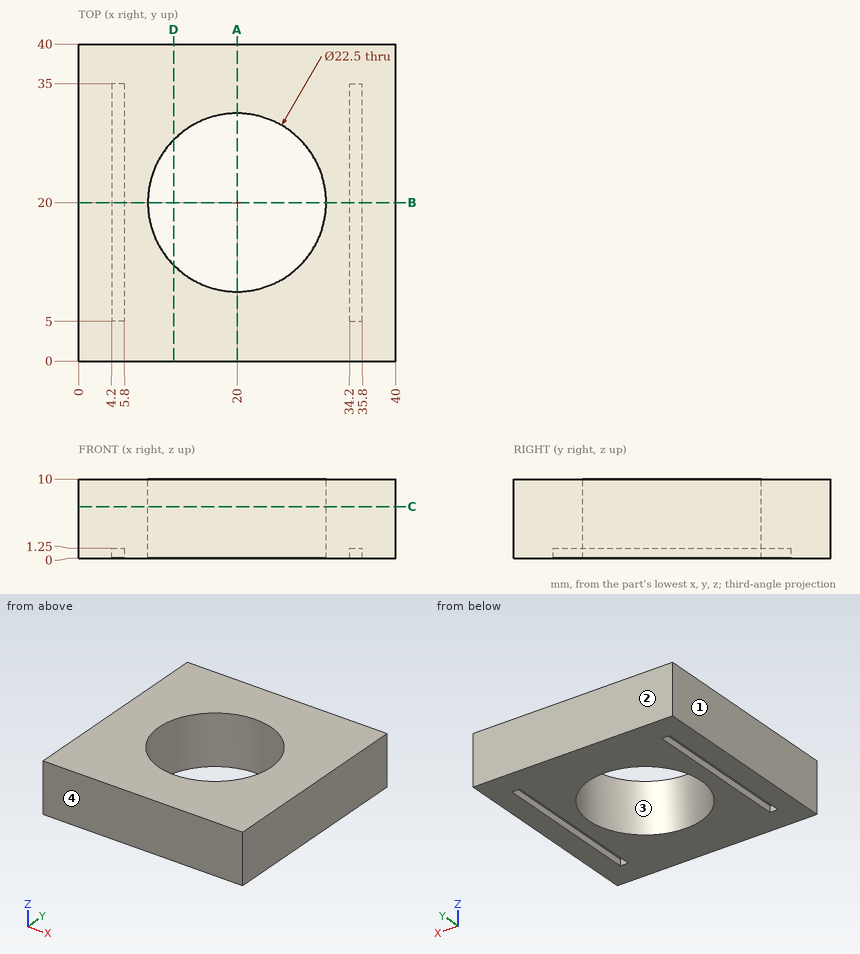
Design review of the part shown in the three views and the two pictorial views. Dimensions are in mm from the part's minimum x, y and z. Coordinates: 2 decimals unless noted, no trailing zeros. Loops run counter-clockwise (first coordinate to the right, second up) from the corner with the lowest first, then second, coordinate; pieces in that order, holes last. Notation, with made-up numbers: (-15.75, 39) -> (13.25, 39) arc R20 cw to (13.25, 45) -> close; hole circle Ø1 at (-16.75, 81.5). An arc over 180 degrees is marked (long way). Answer as CSV lines item,"result".
Item 1: Take a section at B-B, the plane y = 20. State the section outline as (x, z) points.
Results below:
outline,"(0, 0) -> (4.2, 0) -> (4.2, 1.25) -> (5.8, 1.25) -> (5.8, 0) -> (8.75, 0) -> (8.75, 10) -> (0, 10) -> close; (31.25, 0) -> (34.2, 0) -> (34.2, 1.25) -> (35.8, 1.25) -> (35.8, 0) -> (40, 0) -> (40, 10) -> (31.25, 10) -> close"
Item 2: Take a section at A-A, the plane x = 20. State the section outline as (y, z) points, and give its area (3 significant figures).
Results below:
outline,"(0, 0) -> (8.75, 0) -> (8.75, 10) -> (0, 10) -> close; (31.25, 0) -> (40, 0) -> (40, 10) -> (31.25, 10) -> close"
area,"175 mm2"
Item 3: Take a section at D-D, the plane x = 12. State the section outline as (y, z) points.
Results below:
outline,"(0, 0) -> (12.09, 0) -> (12.09, 10) -> (0, 10) -> close; (27.91, 0) -> (40, 0) -> (40, 10) -> (27.91, 10) -> close"
Item 4: For L1, parallel to Y at x = 20, z = 4; L2, parallel to X at y = 22.5, z = 0.75; L3, parallel to Y at x = 17, z = 8.25, list the stretches that pass through material, from the lowest coordinate up.
Results below:
L1,"y = 0 to 8.75, 31.25 to 40"
L2,"x = 0 to 4.2, 5.8 to 9.03, 30.97 to 34.2, 35.8 to 40"
L3,"y = 0 to 9.16, 30.84 to 40"
Item 5: Take a section at C-C, the plane z = 6.5. State the section outline as (x, y) points, and give its area (3 significant figures).
Results below:
outline,"(0, 0) -> (40, 0) -> (40, 40) -> (0, 40) -> close; hole circle Ø22.5 at (20, 20)"
area,"1,200 mm2"
Item 6: Insertion check: pin 1 (0.5 mm diameter, centred on x = 35, y = 22, fed in from -Z). The pin has a flat end and moves straight along its axis. Give the tip position at first contact, or say it passes through.
Results below:
pin 1,"stops at z = 1.25"
Item 7: Draft analysis for pull direction Y (two halves, no side actions). For the marked faces 1, 2, 3 and 4, state which applies: +Y half, -Y half, draft (parallel to the pull), parting line (faces both ways), or undercut.
Results below:
face 1,"draft"
face 2,"+Y half"
face 3,"undercut"
face 4,"-Y half"
